from build123d import *
from OCP.BRepFilletAPI import BRepFilletAPI_MakeChamfer

# Parameters (mm, degrees)
SKETCH_1_W           = 44
SKETCH_1_H           = 34
EXTRUDE_1_DEPTH      = 24
CUT_EXTRUDE_1_DEPTH  = 31
SKETCH_5_W           = 23
SKETCH_5_H           = 9
EXTRUDE_4_DEPTH      = 8
EXTRUDE_5_DEPTH      = 23
SKETCH_7_R           = 1.8
CUT_EXTRUDE_2_DEPTH  = 23
CUT_EXTRUDE_4_DEPTH  = 19
CUT_EXTRUDE_6_REACH  = 62.285
CHAMFER_2_SIZE       = 2
CHAMFER_2_SIZE_2     = 3
SKETCH_11_R          = 1.7
EXTRUDE_6_DEPTH      = 20
CUT_EXTRUDE_7_DEPTH  = 4
CHAMFER_3_SIZE       = 2.4
SKETCH_14_W          = 40.8
SKETCH_14_H          = 4
CUT_EXTRUDE_8_DEPTH  = 18
SKETCH_15_W          = 44
SKETCH_15_H          = 1
CUT_EXTRUDE_9_DEPTH  = 24
SKETCH_16_W          = 3.2
SKETCH_16_H          = 13.6
CUT_EXTRUDE_10_DEPTH = 5
SKETCH_17_W          = 1.6
SKETCH_17_H          = 4
CUT_EXTRUDE_11_DEPTH = 7.4
EXTRUDE_7_DEPTH      = 2
CHAMFER_4_SIZE       = 2


with BuildPart() as part:
    # Sketch 1 → Extrude 1 (new body)
    with BuildSketch(Plane.XY):
        with Locations((0, 27)):
            Rectangle(SKETCH_1_W, SKETCH_1_H)
    extrude(amount=EXTRUDE_1_DEPTH)

    # Sketch 2 → Cut-Extrude 1 (cut)
    with BuildSketch(Plane(origin=(0, 44, 0), x_dir=(1, 0, 0), z_dir=(0, 1, 0))):
        Polygon((-18.8, 0), (18.8, 0), (18.8, -20), (20.4, -20), (20.4, -22), (18.8, -22), (18.8, -24), (-18.8, -24), (-18.8, -22), (-20.4, -22), (-20.4, -20), (-18.8, -20), align=None)
    extrude(amount=-CUT_EXTRUDE_1_DEPTH, mode=Mode.SUBTRACT)



with BuildPart() as body_2:
    # Sketch 5 → Extrude 4 (new body)
    with BuildSketch(Plane(origin=(0, 0, 0), x_dir=(-1, 0, 0), z_dir=(0, 0, -1))):
        with Locations((0, 5.5)):
            Rectangle(SKETCH_5_W, SKETCH_5_H)
    extrude(amount=EXTRUDE_4_DEPTH)


with BuildPart() as part_1:
    add(part.part)

    add(body_2.part)  # Extrude 5 merges body 2
    # Sketch 6 → Extrude 5 (add)
    with BuildSketch(Plane(origin=(11.5, 0, 0), x_dir=(0, 0, -1), z_dir=(1, 0, 0))):
        Polygon((0, 1), (-24, 10), (0, 10), align=None)
    extrude(amount=-EXTRUDE_5_DEPTH)

    # Sketch 7 → Cut-Extrude 2 (cut)
    with BuildSketch(Plane.ZY.offset(11.5)):
        with Locations(Location((-4.5, 5, 0), (0, 0, 270))):
            Circle(SKETCH_7_R)
    extrude(amount=-CUT_EXTRUDE_2_DEPTH, mode=Mode.SUBTRACT)

    # Sketch 8 → Cut-Extrude 4 (cut)
    with BuildSketch(Plane.ZY.offset(9.5)):
        Polygon((0, 10), (20, 13), (0, 13), align=None)
    extrude(amount=-CUT_EXTRUDE_4_DEPTH, mode=Mode.SUBTRACT)

    # Cut-Extrude 6: up to this face of the body (flat: up to its plane)
    cut_extrude_6_end = Plane(part_1.part.faces().sort_by_distance((11.5, 6.483913321, 3.661523268))[0])
    # Sketch 9 → Cut-Extrude 6 (cut, up to the picked face)
    with BuildSketch(Plane.ZY.offset(11.5), mode=Mode.PRIVATE) as cut_extrude_6_sk1:
        Polygon((0, 10), (-8, 7.4), (-8, 10), align=None)
    cut_extrude_6_tool1 = split(extrude(cut_extrude_6_sk1.sketch, amount=-CUT_EXTRUDE_6_REACH, mode=Mode.PRIVATE), bisect_by=cut_extrude_6_end, keep=Keep.BOTH, mode=Mode.PRIVATE)
    add(cut_extrude_6_tool1.solids().sort_by(Axis((-11.5, 9.133333, -5.333333), (1, 0, 0)))[0], mode=Mode.SUBTRACT)

    # Chamfer 2
    chamfer_2_edges_1 = [part_1.edges().sort_by_distance(p)[0] for p in [
        (-9.5, 13, 10),
    ]]
    chamfer_2_side_1 = [part_1.faces().sort_by_distance(p)[0] for p in [
        (-9.54, 13, 10),
    ]]
    chamfer_2_edges_2 = [part_1.edges().sort_by_distance(p)[0] for p in [
        (9.5, 13, 10),
    ]]
    chamfer_2_side_2 = [part_1.faces().sort_by_distance(p)[0] for p in [
        (9.5, 12.96, 10),
    ]]
    chamfer_2 = BRepFilletAPI_MakeChamfer(part_1.part.solid().wrapped)
    for e in chamfer_2_edges_1:
        chamfer_2.Add(CHAMFER_2_SIZE - 0.0001, CHAMFER_2_SIZE_2 - 0.0001, e.wrapped, chamfer_2_side_1[0].wrapped)
    for e in chamfer_2_edges_2:
        chamfer_2.Add(CHAMFER_2_SIZE_2 - 0.0001, CHAMFER_2_SIZE - 0.0001, e.wrapped, chamfer_2_side_2[0].wrapped)
    add(Compound.cast(chamfer_2.Shape()), mode=Mode.REPLACE)  # a hair under: the kernel refuses the full size

    # Sketch 11 → Extrude 6 (add)
    # profile 1 of 2: a face of its own
    with BuildSketch(Plane(origin=(0, 0, 0), x_dir=(-1, 0, 0), z_dir=(0, 0, -1))):
        with BuildLine():
            Line((-14, 43), (-18.8, 43))
            Line((-18.8, 43), (-18.8, 35.6))
            Line((-18.8, 35.6), (-14, 35.6))
            ThreePointArc((-14, 35.6), (-10.3, 39.3), (-14, 43))
        make_face()
        with Locations((-14, 39.3)):
            Circle(SKETCH_11_R, mode=Mode.SUBTRACT)
    # profile 2 of 2: a face of its own
    with BuildSketch(Plane(origin=(0, 0, 0), x_dir=(-1, 0, 0), z_dir=(0, 0, -1))):
        with BuildLine():
            Line((18.8, 35.6), (14, 35.6))
            ThreePointArc((14, 35.6), (10.3, 39.3), (14, 43))
            Line((14, 43), (18.8, 43))
            Line((18.8, 43), (18.8, 35.6))
        make_face()
        with Locations((14, 39.3)):
            Circle(SKETCH_11_R, mode=Mode.SUBTRACT)
    extrude(amount=-EXTRUDE_6_DEPTH)

    # Sketch 13 → Cut-Extrude 7 (cut)
    with BuildSketch(Plane.ZY.offset(22)):
        Polygon((2, 34), (17, 36), (17, 34), (2, 32), align=None)
        Polygon((2, 30), (17, 32), (17, 30), (2, 28), align=None)
        Polygon((2, 26), (17, 28), (17, 26), (2, 24), align=None)
        Polygon((2, 22), (17, 24), (17, 22), (2, 20), align=None)
        Polygon((2, 18), (17, 20), (17, 18), (2, 16), align=None)
    cut_extrude_7 = extrude(amount=-CUT_EXTRUDE_7_DEPTH, mode=Mode.SUBTRACT)

    # Mirror 1: Cut-Extrude 7 across plane
    add(cut_extrude_7.mirror(Plane(origin=(0, 0, 0), x_dir=(0, 0, 1), z_dir=(1, 0, 0))), mode=Mode.SUBTRACT)

    # Chamfer 3
    chamfer_3_edges = [part_1.edges().sort_by_distance(p)[0] for p in [
        (22, 10, 12),
        (-22, 10, 12),
    ]]
    chamfer(chamfer_3_edges, length=CHAMFER_3_SIZE)

    # Sketch 14 → Cut-Extrude 8 (cut)
    with BuildSketch(Plane(origin=(0, 44, 0), x_dir=(1, 0, 0), z_dir=(0, 1, 0))):
        with Locations((0, -22)):
            Rectangle(SKETCH_14_W, SKETCH_14_H)
    extrude(amount=-CUT_EXTRUDE_8_DEPTH, mode=Mode.SUBTRACT)

    # Sketch 15 → Cut-Extrude 9 (cut)
    with BuildSketch(Plane(origin=(0, 0, 0), x_dir=(-1, 0, 0), z_dir=(0, 0, -1))):
        with Locations((0, 43.5)):
            Rectangle(SKETCH_15_W, SKETCH_15_H)
    extrude(amount=-CUT_EXTRUDE_9_DEPTH, mode=Mode.SUBTRACT)

    # Sketch 16 → Cut-Extrude 10 (cut)
    with BuildSketch(Plane.XY.offset(24)):
        with Locations((20.4, 28.8)):
            Rectangle(SKETCH_16_W, SKETCH_16_H)
    extrude(amount=-CUT_EXTRUDE_10_DEPTH, mode=Mode.SUBTRACT)

    # Sketch 17 → Cut-Extrude 11 (cut)
    with BuildSketch(Plane(origin=(0, 43, 0), x_dir=(1, 0, 0), z_dir=(0, 1, 0))):
        with Locations((21.2, -22)):
            Rectangle(SKETCH_17_W, SKETCH_17_H)
    extrude(amount=-CUT_EXTRUDE_11_DEPTH, mode=Mode.SUBTRACT)

    # Sketch 18 → Extrude 7 (add)
    with BuildSketch(Plane(origin=(0, 0, 0), x_dir=(-1, 0, 0), z_dir=(0, 0, -1))):
        Polygon((-22, 43), (-18.8, 43), (-18.8, 10), (-19.6, 10), (-22, 12.4), align=None)
        Polygon((22, 12.4), (19.6, 10), (18.8, 10), (18.8, 43), (22, 43), align=None)
    extrude(amount=EXTRUDE_7_DEPTH)

    # Chamfer 4
    chamfer_4_edges = [part_1.edges().sort_by_distance(p)[0] for p in [
        (-20.4, 43, -2),
        (20.4, 43, -2),
    ]]
    chamfer(chamfer_4_edges, length=CHAMFER_4_SIZE)


solid = part_1.part
Input: part model. Units: mm. Frame: model coordinates. A direction names the side the tool comes from. Coordinates: 2 decimals unless noted, no trailing zeros. Order: outer loops, then holes, each group sorted by start corner. A loop starts at its lowest first (then second) coordinate and runs counter-clockwise, first axis right, second up. Notation, with made-up numbers: M 18,-20 L 75,-20 A3 cw 75,-16 Z; hole C 24.5,63 d1. An arc over 180 degrees is marked long. Answer in a Markdown table with one row per item.
(1) Access query for faces 5 (the flat face through (-20, 23, 17)), 6 (the flat face through (-14, 12, 0)), 7 (the flat face through (0, 4, -8)). Directions: +Z, -Z, +X, -X, +Y, -Y. A direction counts if a zero-diameter tool reaches every point of the face in a straight line with its end or side. Return the directions, or none.
Numbers:
| item | result |
|---|---|
| face 5 | +X, -X |
| face 6 | -Z, +Y |
| face 7 | -Z, +X, -X, +Y, -Y |
(2) Section query A-A, the plane y = 39.3. Output: boundary loops of the cut face in (x, z).
Numbers:
| item | result |
|---|---|
| outline | M -22,-2 L -18.8,-2 L -18.8,0 L -15.7,0 L -15.7,20 L -20.4,20 L -20.4,24 L -22,24 Z; M -12.3,0 L -10.3,0 L -10.3,20 L -12.3,20 Z; M 10.3,0 L 12.3,0 L 12.3,20 L 10.3,20 Z; M 15.7,0 L 18.8,0 L 18.8,-2 L 22,-2 L 22,20 L 15.7,20 Z |
(3) Section query D-D, the plane y = 5. Output: boundary loops of the cut face in (x, z), plus the area to 3 significant figures.
Numbers:
| item | result |
|---|---|
| outline | M -11.5,-8 L 11.5,-8 L 11.5,-6.3 L -11.5,-6.3 Z; M -11.5,-2.7 L 11.5,-2.7 L 11.5,10.67 L -11.5,10.67 Z |
| area | 347 mm^2 |
(4) Section query B-B, the plane z = -4.5. Output: boundary loops of the cut face in (x, y), plus the area to 3 significant figures.
Numbers:
| item | result |
|---|---|
| outline | M -11.5,1 L 11.5,1 L 11.5,3.2 L -11.5,3.2 Z; M -11.5,6.8 L 11.5,6.8 L 11.5,8.54 L -11.5,8.54 Z |
| area | 90.6 mm^2 |
(5) Section query C-C, the plane x = 15. Output: boundary loops of the cut face in (y, z), plus the area to 3 significant figures.
Numbers:
| item | result |
|---|---|
| outline | M 10,0 L 13,0 L 13,24 L 10,24 Z; M 35.6,0 L 37.93,0 L 37.93,20 L 35.6,20 Z; M 40.67,0 L 43,0 L 43,20 L 40.67,20 Z |
| area | 165 mm^2 |
(6) Contact query for flat-ended pins moving along their axis: pin 1 Ø0.5 at (x, z) = (-20, 23) entering from +Y; pin 2 Ø0.6 at (x, y) = (20, 19.5) entering from -Z; pin 3 Ø0.6 at (x, y) = (20, 28.5) entering from +Z; pin 4 Ø3 at (y, z) = (5, -4.5) entering from +X. Output: stop coordinate, or through.
Numbers:
| item | result |
|---|---|
| pin 1 | stops at y = 26 |
| pin 2 | stops at z = -2 |
| pin 3 | stops at z = 19 |
| pin 4 | passes through |
(7) Material intervals for line 1 (Y direction, x = 14, z = 9); line 2 (Y direction, x = -19, z = 15); line 3 (Y direction, x = 18.5, z = 7), sorted ascending. Write a range as [from, to].
Numbers:
| item | result |
|---|---|
| line 1 | y = [10, 13], [35.6, 37.6], [41, 43] |
| line 2 | y = [10, 17.73], [19.73, 21.73], [23.73, 25.73], [27.73, 29.73], [31.73, 33.73], [35.73, 43] |
| line 3 | y = [10, 13], [35.6, 43] |
(8) Draft query along Y for faces 1 (the cylindrical face through (-10.3, 39.2, 9.9)), 2 (the flat face through (0, 1, -4)), 3 (the flat face through (16, 39, 0)), 4 (the flat face through (20, 23, 17)). Return one class per face: pulls with the +Y half, pulls with the -Y half, needs draft (parallel to the pull), parting line crosses it, or undercut.
Numbers:
| item | result |
|---|---|
| face 1 | undercut |
| face 2 | pulls with the -Y half |
| face 3 | needs draft |
| face 4 | undercut |
